The listing builds one solid part. Answer for the finished solid, in the listing's coordinates (mm). Face numbers are marked on the shaded views. Round coordinates to 2 decimals unless told otherwise and drop trailing zeros. Order: outer loops, then holes, each group sorted by start corner. A loop starts at its lowest first (then second) coordinate and runs counter-clockwise, first axis right, second up. Notation, with made-up numbers: (72.25, 76.5) -> (82.25, 76.5) arc R32 ccw to (82.25, 110.5) -> close; hole circle Ø5 at (36.25, 65). An arc over 180 degrees is marked (long way). Return JSON: item names as keys, results as strings. Group by question number.
(1) The part is cut by section C-C (z = -60). Determine the outline of the cut face in (x, y), plus the area to 3 significant figures.
(2) The part is cut by section A-A (z = -200). Determine the outline of the cut face in (x, y), plus the area to 3 significant figures.
(3) The part is cut by section B-B (x = 541.5). Determine the outline of the cut face in (y, z), plus the area to 3 significant figures.
(4) Each of these flat-tipped pins is pushed along its axis until it touches: pin 1 (12.5 mm diameter, centred on x = 330.5, y = -9.5, fed in from +Z); pin 2 (6 mm diameter, centred on x = 440, z = -275, fed in from -Y); pin 3 (2 mm diameter, centred on x = 181, z = -391.5, fed in from -Y). Where does it stop, or does it pass through?
(5) The part is cut by section D-D (x = 717.5). Determine the outline of the cut face in (y, z).
(6) Consider line 1 (X direction, y = -30.5, z = -42.5); line 2 (Y direction, x = 616.5, z = -583.5); line 3 (X direction, y = -34.5, z = -69). Determine where each line is inside the solid, lowest interval first. Write a range as [from, to].
(7) Determine the mould class of the marked faces 1 and 2 for opening direction Z: +Z half, -Z half, draft (parallel to the pull), parting line (faces both ways), or undercut.
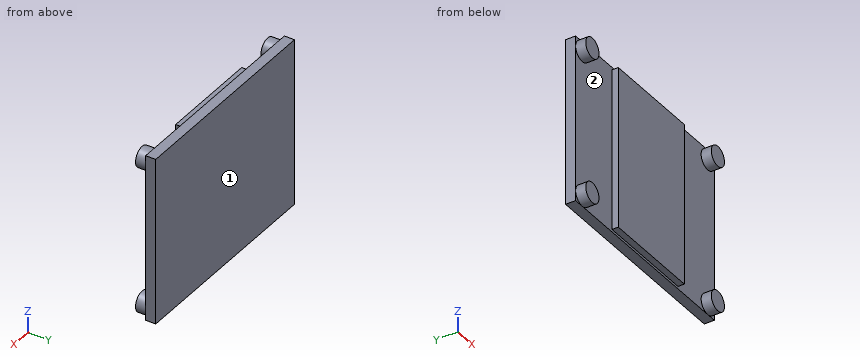
from build123d import *

# Parameters (mm, degrees)
SKETCH1_W           = 840
SKETCH1_H           = 660
BOSS_EXTRUDE1_DEPTH = 40
SKETCH2_R           = 40
BOSS_EXTRUDE2_DEPTH = 40
SKETCH3_W           = 400
SKETCH3_H           = 640
BOSS_EXTRUDE3_DEPTH = 25


with BuildPart() as part:
    # Sketch1 → Boss-Extrude1 (new body)
    with BuildSketch(Plane(origin=(0, 0, 0), x_dir=(1, 0, 0), z_dir=(0, 1, 0))):
        with Locations((420, 330)):
            Rectangle(SKETCH1_W, SKETCH1_H)
    extrude(amount=BOSS_EXTRUDE1_DEPTH)

    # Sketch2 → Boss-Extrude2 (add)
    with BuildSketch(Plane.XZ):
        with Locations(Location((40, -40, 0), (0, 0, 90))):
            Circle(SKETCH2_R)
        with Locations(Location((800, -40, 0), (0, 0, 90))):
            Circle(SKETCH2_R)
        with Locations(Location((40, -620, 0), (0, 0, 270))):
            Circle(SKETCH2_R)
        with Locations(Location((800, -620, 0), (0, 0, 270))):
            Circle(SKETCH2_R)
    extrude(amount=BOSS_EXTRUDE2_DEPTH)

    # Sketch3 → Boss-Extrude3 (add)
    with BuildSketch(Plane.XZ):
        with Locations((420, -330)):
            Rectangle(SKETCH3_W, SKETCH3_H)
    extrude(amount=BOSS_EXTRUDE3_DEPTH)


solid = part.part
Answer below:
{
 "1": {"outline": "(0, 0) -> (5.36, 0) -> (5.36, -40) -> (74.64, -40) -> (74.64, 0) -> (220, 0) -> (220, -25) -> (620, -25) -> (620, 0) -> (765.36, 0) -> (765.36, -40) -> (834.64, -40) -> (834.64, 0) -> (840, 0) -> (840, 40) -> (0, 40) -> close", "area": "49,100 mm²"},
 "2": {"outline": "(0, 0) -> (220, 0) -> (220, -25) -> (620, -25) -> (620, 0) -> (840, 0) -> (840, 40) -> (0, 40) -> close", "area": "43,600 mm²"},
 "3": {"outline": "(-25, -650) -> (0, -650) -> (0, -660) -> (40, -660) -> (40, 0) -> (0, 0) -> (0, -10) -> (-25, -10) -> close", "area": "42,400 mm²"},
 "4": {"pin 1": "stops at z = -10", "pin 2": "stops at y = -25", "pin 3": "stops at y = 0"},
 "5": {"outline": "(0, -660) -> (40, -660) -> (40, 0) -> (0, 0) -> close"},
 "6": {"line 1": "x = [0.08, 79.92], [760.08, 839.92]", "line 2": "y = [-25, 40]", "line 3": "x = [12.45, 67.55], [772.45, 827.55]"},
 "7": {"face 1": "draft", "face 2": "undercut"}
}
